Solid Edge part; units mm, degrees
sketch "Sketch1" plane through (0, 0, 0) normal (0, -1, 0) x (1, 0, 0)
  arc A0 (-5.5, 23.1) -> (-10.4, 18.2) centre (-5.5, 18.2) ccw
  line L0 (-10.4, 18.2) -> (-10.4, 18)
  arc A1 (-10.4, 18) -> (-5.5, 13.1) centre (-5.5, 18) ccw
  line L1 (-5.5, 13.1) -> (25.4, 13.1)
  line L2 (25.4, 13.1) -> (25.4, -38.1)
  line L3 (25.4, -38.1) -> (-25.4, -38.1)
  line L4 (-25.4, -38.1) -> (-25.4, -23.1)
  line L5 (5.5, -23.1) -> (-25.4, -23.1)
  arc A2 (10.4, -18.2) -> (5.5, -23.1) centre (5.5, -18.2) cw
  line L6 (10.4, -18) -> (10.4, -18.2)
  arc A3 (5.5, -13.1) -> (10.4, -18) centre (5.5, -18) cw
  line L7 (-25.4, -13.1) -> (5.5, -13.1)
  line L8 (-25.4, -13.1) -> (-25.4, 38.1)
  line L9 (-25.4, 38.1) -> (25.4, 38.1)
  line L10 (25.4, 38.1) -> (25.4, 23.1)
  line L11 (25.4, 23.1) -> (-5.5, 23.1)
extrude "Protrusion1" add sketch "Sketch1" against normal blind 19
sketch "Sketch2" plane through (0, 9.5, 38.1) normal (0, 0, 1) x (-1, 0, 0)
  circle A0 centre (0, 0) radius 6
extrude "Cutout1" cut sketch "Sketch2" against normal through all
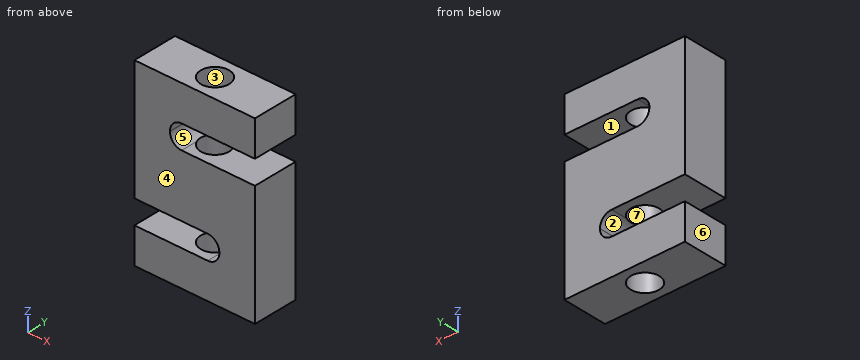
CAD build for the part. Positions are in the model's coordinates, mm. Face numbers are marked on the shaded views. A direction names the side the tool comes from. Round coordinates to 2 decimals unless told otherwise and drop trailing zeros. Order: outer loops, then holes, each group sorted by start corner. A loop starts at its lowest first (then second) coordinate and runs counter-clockwise, first axis right, second up.
Item 1: Pin check, flat tips, straight feed: pin 1 (11 mm diameter, centred on x = 0, y = 9.5, fed in from -Z); pin 2 (6 mm diameter, centred on x = -16, z = -27.5, fed in from -Y). Stop position of each tip, or through.
Item 2: Saw through at B-B on y = 9.5. Write the cut outline in (x, z).
Item 3: Tool access for the marked faces 1, 2 and 3: list every direction of +Z, -Z, +X, -X, +Y, -Y with a clear straight run to the whole face (end or side of a thin tool).
Item 4: Saw through at D-D on z = -33. Write the cut outline in (x, y).
Item 5: Saw through at C-C on x = 12. Write the cut outline in (y, z), then the cut area to 3 significant figures.
Item 6: Mould opens along X. For the marked faces 4, 5, 6 and 7 say: pulls with the +X half, pulls with the -X half, needs draft (parallel to the pull), parting line crosses it, or undercut.
Item 7: Probe line 1 along Z through (x, y) = (-4.5, 1.5); line 2 along Y through (x, z) = (0, 32); line 3 along Z through (x, y) = (23, 14.25). List the from-to ranges inside material, lowest first.
Item 8: Saw through at A-A on x = 0. Write the cut outline in (y, z).
Reported:
1. pin 1: passes through
1. pin 2: stops at y = 0
2. outline: (-25.4, -38.1) - (-6, -38.1) - (-6, -23.1) - (-25.4, -23.1) - close; (-25.4, -13.1) - (-6, -13.1) - (-6, 13.13) arc R4.9 cw to (-10.4, 18) - (-10.4, 18.2) arc R4.9 cw to (-6, 23.07) - (-6, 38.1) - (-25.4, 38.1) - close; (6, -38.1) - (25.4, -38.1) - (25.4, 13.1) - (6, 13.1) - (6, -13.13) arc R4.9 cw to (10.4, -18) - (10.4, -18.2) arc R4.9 cw to (6, -23.07) - close; (6, 23.1) - (25.4, 23.1) - (25.4, 38.1) - (6, 38.1) - close
3. face 1: +X, +Y, -Y
3. face 2: -X, +Y, -Y
3. face 3: +Z, -Z
4. outline: (-25.4, 0) - (25.4, 0) - (25.4, 19) - (-25.4, 19) - close; hole circle Ø12 at (0, 9.5)
5. outline: (0, -38.1) - (19, -38.1) - (19, 13.1) - (0, 13.1) - close; (0, 23.1) - (19, 23.1) - (19, 38.1) - (0, 38.1) - close
5. area: 1,260 mm2
6. face 4: needs draft
6. face 5: pulls with the +X half
6. face 6: pulls with the -X half
6. face 7: undercut
7. line 1: z = -38.1 to -23.1, -13.1 to 13.1, 23.1 to 38.1
7. line 2: y = 0 to 3.5, 15.5 to 19
7. line 3: z = -38.1 to 13.1, 23.1 to 38.1
8. outline: (0, -38.1) - (3.5, -38.1) - (3.5, -23.1) - (0, -23.1) - close; (0, -13.1) - (3.5, -13.1) - (3.5, 13.1) - (0, 13.1) - close; (0, 23.1) - (3.5, 23.1) - (3.5, 38.1) - (0, 38.1) - close; (15.5, -38.1) - (19, -38.1) - (19, -23.1) - (15.5, -23.1) - close; (15.5, -13.1) - (19, -13.1) - (19, 13.1) - (15.5, 13.1) - close; (15.5, 23.1) - (19, 23.1) - (19, 38.1) - (15.5, 38.1) - close
